Input: part model. Units: mm. Frame: model coordinates. A direction names the side the tool comes from. Give positions to 0.01 mm unless a question says otherwise; leave off trailing zeros. Order: outer loops, then holes, each group sorted by start corner. A loop starts at its lowest first (then second) coordinate and runs counter-clockwise, first axis right, second up. Notation, with made-up numbers: (81.5, -7) - (97.5, -7) arc R18 ccw to (97.5, 1) - close; hole circle Ø10 at (59, 73.5). An arc over 180 degrees is marked (long way). Answer in a Markdown table with one row per item. Add a question column.
1. Section query B-B on x = 25. Return loops of the section in (y, z).
2. Access query for faces 1 (the face through (54.612, -8.28, -37.353)), 2 (the face through (-44, -2, 50.8)), 3 (the face through (-62, -12.878, -36)). Directions: +Z, -Z, +X, -X, +Y, -Y. A direction counts if a zero-diameter tool reaches every point of the face in a straight line with its end or side. Return the directions, or none.
3. Section query A-A on y = -34. Return loops of the section in (x, z) (3 decimals), and give its area (3 significant figures).
4. Section query D-D on x = -23. Return loops of the section in (y, z) (3 decimals), and give its area (3 significant figures).
5. Section query C-C on z = 6.5. Return loops of the section in (x, y).
6. Ray query, line 1 (Z direction, x = -62, y = -8); line 2 (X direction, y = -119, z = -3); line 3 (X direction, y = -25, z = 25). Return the intervals inside material, ascending. Write a range as [from, to].
7. Mould query, pull axis X, two halves, no side actions, for faces 4 (the face through (99.06, -64, -1)), 5 (the face through (55.134, -8.28, 35.919)), 6 (the face through (-1, -3.81, 1)), 7 (the face through (-99.06, -64, -1)). Classes: released by +X, released by -X, zero draft, split by the parting line, or undercut.
8. Contact query for flat-ended pins moving along their axis: pin 1 (3 mm diameter, centred on x = 57.5, z = -37.5, fed in from -Y); pin 2 (1.3 mm diameter, centred on x = -62.5, z = 37.5, fed in from -Y). Output: stop coordinate, or through.
```python
from build123d import *

# Parameters (mm, degrees)
F0_W      = 198.12
F0_H      = 101.6
F2_DEPTH  = 3.81
F1_R      = 2.54
F3_DEPTH  = 12.8778
F4_R      = 1.2742822285
F4_R_2    = 1.2649039603
F4_R_3    = 1.2682976719
F4_R_4    = 1.273443292
F4_R_5    = 1.26744028
F4_R_6    = 1.2643596857
F5_DEPTH  = 10.3378
F6_W      = 54.61
F6_H      = 71.882
F6_W_2    = 1.524
F6_H_2    = 1.524
F7_DEPTH  = 3.81
F8_W      = 3.81
F8_H      = 101.6
F9_DEPTH  = 127
F10_W     = 2.54
F10_H     = 2.54
F10_H_2   = 2.5507584214
F10_R     = 1.2654265937
F10_R_2   = 1.2754683581
F10_R_3   = 1.268876748
F10_R_4   = 1.2699045753
F11_DEPTH = 127


with BuildPart() as f2:
    # F0 (on Front) → F2 (new body)
    with BuildSketch(Plane.XZ):
        Rectangle(F0_W, F0_H)
    extrude(amount=F2_DEPTH)

    # F1 (on Front) → F3 (join)
    with BuildSketch(Plane.XZ):
        with Locations((-62.23, -37.465)):
            Circle(F1_R)
        with Locations((-62.23, 37.465)):
            Circle(F1_R)
        with Locations((0, 37.465)):
            Circle(F1_R)
        with Locations((0, -37.465)):
            Circle(F1_R)
        with Locations((57.15, -37.465)):
            Circle(F1_R)
        with Locations((57.15, 37.465)):
            Circle(F1_R)
    extrude(amount=F3_DEPTH)

    # F4 (on face) → F5 (cut)
    with BuildSketch(Plane.XZ.offset(3.81)):
        with Locations((-62.23, 37.465)):
            Circle(F4_R)
        with Locations((-62.23, -37.465)):
            Circle(F4_R_2)
        with Locations((57.15, -37.465)):
            Circle(F4_R_3)
        with Locations((57.15, 37.465)):
            Circle(F4_R_4)
        with Locations((0, -37.465)):
            Circle(F4_R_5)
        with Locations((0, 37.465)):
            Circle(F4_R_6)
    extrude(amount=F5_DEPTH, mode=Mode.SUBTRACT)

    # F6 (on face) → F7 (cut)
    with BuildSketch(Plane.XZ.offset(3.81)):
        with Locations((-31.115, 1.524)):
            Rectangle(F6_W, F6_H)
        with BuildLine():
            ThreePointArc((15.9514440232, -2.413179692), (8.8903213435, -9.5926068587), (16.086657352, -16.6364961248))
            Line((16.086657352, -16.6364961248), (41.317342648, -16.6364961248))
            ThreePointArc((41.317342648, -16.6364961248), (34.29, -9.525), (41.317342648, -2.4135038752))
            Line((41.317342648, -2.4135038752), (41.317342648, -2.413179692))
            Line((41.317342648, -2.413179692), (15.9514440232, -2.413179692))
        make_face()
        with BuildLine():
            ThreePointArc((15.9514440232, -2.413179692), (21.0130373124, -4.4782139877), (23.114, -9.525))
            ThreePointArc((23.114, -9.525), (21.0607857776, -14.5239229296), (16.086657352, -16.6364961248))
            Line((16.086657352, -16.6364961248), (15.9514440232, -16.6364961248))
            Line((15.9514440232, -16.6364961248), (15.9514440232, -2.413179692))
        make_face(mode=Mode.SUBTRACT)
        with BuildLine():
            Line((41.317342648, -2.4135038752), (41.317342648, -16.6364961248))
            ThreePointArc((41.317342648, -16.6364961248), (46.4009229296, -14.5837857776), (48.514, -9.525))
            ThreePointArc((48.514, -9.525), (46.4009229296, -4.4662142224), (41.317342648, -2.4135038752))
        make_face()
        with BuildLine():
            ThreePointArc((16.086657352, -16.6364961248), (21.0607857776, -14.5239229296), (23.114, -9.525))
            ThreePointArc((23.114, -9.525), (21.0130373124, -4.4782139877), (15.9514440232, -2.413179692))
            Line((15.9514440232, -2.413179692), (15.9514440232, -16.6364961248))
            Line((15.9514440232, -16.6364961248), (16.086657352, -16.6364961248))
        make_face()
        with BuildLine():
            ThreePointArc((41.317342648, -2.4135038752), (34.29, -9.525), (41.317342648, -16.6364961248))
            Line((41.317342648, -16.6364961248), (41.317342648, -2.4135038752))
        make_face()
        with Locations((28.702, 9.525)):
            Rectangle(F6_W_2, F6_H_2)
    extrude(amount=-F7_DEPTH, mode=Mode.SUBTRACT)

    # F8 (on face) → F9 (join)
    with BuildSketch(Plane.XZ.offset(3.81)):
        with Locations((-97.155, 0)):
            Rectangle(F8_W, F8_H)
        with Locations((97.155, 0)):
            Rectangle(F8_W, F8_H)
    extrude(amount=F9_DEPTH)

    # F10 (on face) → F11 (cut)
    with BuildSketch(Plane.XZ.offset(3.81)):
        with Locations((-96.52, 46.99)):
            Rectangle(F10_W, F10_H)
        with Locations((-96.52, -46.9846207893)):
            Rectangle(F10_W, F10_H_2)
        with Locations((96.52, 46.99)):
            Rectangle(F10_W, F10_H)
        with Locations((96.52, -46.99)):
            Rectangle(F10_W, F10_H)
        with Locations((97.155, -25.4)):
            Circle(F10_R)
        with Locations((97.155, 25.4)):
            Circle(F10_R_2)
        with Locations((-97.155, 25.4)):
            Circle(F10_R_3)
        with Locations((-97.155, -25.4)):
            Circle(F10_R_4)
    extrude(amount=F11_DEPTH, mode=Mode.SUBTRACT)


solid = f2.part
```
Answer:
| question | item | result |
|---|---|---|
| 1 | outline | (-3.81, -50.8) - (0, -50.8) - (0, -16.64) - (-3.81, -16.64) - close; (-3.81, -2.41) - (0, -2.41) - (0, 50.8) - (-3.81, 50.8) - close |
| 2 | face 1 | -Y |
| 2 | face 2 | +Z, +X, -X, +Y, -Y |
| 2 | face 3 | +Z, -Z, -Y |
| 3 | outline | (-99.06, -50.8) - (-95.25, -50.8) - (-95.25, -48.26) - (-97.79, -48.26) - (-97.79, -45.709) - (-95.25, -45.709) - (-95.25, 45.72) - (-97.79, 45.72) - (-97.79, 48.26) - (-95.25, 48.26) - (-95.25, 50.8) - (-99.06, 50.8) - close; (95.25, -50.8) - (99.06, -50.8) - (99.06, 50.8) - (95.25, 50.8) - (95.25, 48.26) - (97.79, 48.26) - (97.79, 45.72) - (95.25, 45.72) - (95.25, -45.72) - (97.79, -45.72) - (97.79, -48.26) - (95.25, -48.26) - close; hole circle Ø2.54 at (-97.155, -25.4); hole circle Ø2.538 at (-97.155, 25.4); hole circle Ø2.551 at (97.155, 25.4); hole circle Ø2.531 at (97.155, -25.4) |
| 3 | area | 728 mm² |
| 4 | outline | (-3.81, -50.8) - (0, -50.8) - (0, -34.417) - (-3.81, -34.417) - close; (-3.81, 37.465) - (0, 37.465) - (0, 50.8) - (-3.81, 50.8) - close |
| 4 | area | 113 mm² |
| 5 | outline | (-99.06, -130.81) - (-95.25, -130.81) - (-95.25, -3.81) - (-58.42, -3.81) - (-58.42, 0) - (-99.06, 0) - close; (-3.81, -3.81) - (95.25, -3.81) - (95.25, -130.81) - (99.06, -130.81) - (99.06, 0) - (-3.81, 0) - close |
| 6 | line 1 | z = [-39.99, -38.71], [-36.22, -34.94], [34.94, 36.21], [38.72, 39.99] |
| 6 | line 2 | x = [-99.06, -95.25], [95.25, 99.06] |
| 6 | line 3 | x = [-99.06, -98.36], [-95.95, -95.25], [95.25, 95.94], [98.37, 99.06] |
| 7 | face 4 | released by +X |
| 7 | face 5 | undercut |
| 7 | face 6 | undercut |
| 7 | face 7 | released by -X |
| 8 | pin 1 | stops at y = -12.88 |
| 8 | pin 2 | stops at y = -3.81 |
